from build123d import *

# Parameters (mm, degrees)
F1_DEPTH = 38.1
F2_DEPTH = 6.35
F0_W     = 6.3290558755
F0_H     = 12.5651992857
F3_DEPTH = 3.175
F0_R     = 8.6525424745
F0_R_2   = 9.0711492587
F0_W_2   = 5.1460258761
F0_H_2   = 10.5661942953
F0_W_3   = 24.5602354407
F0_W_4   = 26.5593226068
F0_W_5   = 6.9090700396
F0_W_6   = 14.06177961
F0_W_7   = 3.8753339521
F0_R_3   = 3.8842075561
F4_DEPTH = 25.4


with BuildPart() as f1:
    # F0 (on Front) → F1 (new body, symmetric)
    with BuildSketch(Plane.XZ):
        with BuildLine():
            Line((-51.1175096035, -16.873287037), (-51.1175096035, -22.5602444261))
            Line((-51.1175096035, -22.5602444261), (50.8410625258, -22.5602444261))
            ThreePointArc((50.8410625258, -22.5602444261), (83.7910011304, -14.7143733495), (109.6690327028, 7.1393135004))
            Line((109.6690327028, 7.1393135004), (93.1019932032, 7.1393135004))
            Line((93.1019932032, 7.1393135004), (71.9687715173, 7.1393135004))
            Line((71.9687715173, 7.1393135004), (50.8410625258, 7.1393135004))
            Line((50.8410625258, 7.1393135004), (45.6950366497, 7.1393135004))
            Line((45.6950366497, 7.1393135004), (21.134801209, 7.1393135004))
            Line((21.134801209, 7.1393135004), (-5.4245213978, 7.1393135004))
            Line((-5.4245213978, 7.1393135004), (-12.3335914374, 7.1393135004))
            Line((-12.3335914374, 7.1393135004), (-26.3953710475, 7.1393135004))
            Line((-26.3953710475, 7.1393135004), (-30.2707049996, 7.1393135004))
            Line((-30.2707049996, 7.1393135004), (-51.1175096035, 7.1393135004))
            Line((-51.1175096035, 7.1393135004), (-51.1175096035, 6.1453658742))
            Line((-51.1175096035, 6.1453658742), (-51.1175096035, -16.873287037))
        make_face()
    extrude(amount=F1_DEPTH, both=True)

    # F0 (on Front) → F2 (join, symmetric)
    with BuildSketch(Plane.XZ):
        Polygon((-55.0226159394, -16.873287037), (-51.1175096035, -16.873287037), (-51.1175096035, 6.1453658742), (-71.5858340263, 0), (-71.5858340263, -16.873287037), (-61.3516718149, -16.873287037), align=None)
    extrude(amount=F2_DEPTH, both=True)

    # F0 (on Front) → F3 (join, symmetric)
    with BuildSketch(Plane.XZ):
        with Locations((-58.1871438771, -23.1558866799)):
            Rectangle(F0_W, F0_H)
    extrude(amount=F3_DEPTH, both=True)

    # F0 (on Front) → F4 (join, symmetric)
    with BuildSketch(Plane.XZ):
        with BuildLine():
            Line((-30.2707049996, 50.5518508265), (-30.2707049996, 17.7055077956))
            Line((-30.2707049996, 17.7055077956), (-26.3953710475, 17.7055077956))
            Line((-26.3953710475, 17.7055077956), (-26.3953710475, 42.5316623055))
            add(Edge.make_bspline(
                [(-26.3953710475, 42.5316623055), (-25.6086271256, 50.5518508265), (-13.6145753786, 50.5218580365), (-12.3335914374, 42.5316623055)],
                knots=[0, 0, 0, 0, 14.06177961, 14.06177961, 14.06177961, 14.06177961], degree=3))
            Line((-12.3335914374, 42.5316623055), (-12.3335914374, 17.7055077956))
            Line((-12.3335914374, 17.7055077956), (-5.4245213978, 17.7055077956))
            Line((-5.4245213978, 17.7055077956), (21.134801209, 17.7055077956))
            Line((21.134801209, 17.7055077956), (45.6950366497, 17.7055077956))
            Line((45.6950366497, 17.7055077956), (50.8410625258, 17.7055077956))
            Line((50.8410625258, 17.7055077956), (50.8410625258, 50.5518508265))
            Line((50.8410625258, 50.5518508265), (-30.2707049996, 50.5518508265))
        make_face()
        with Locations((0, 36.2432263792)):
            Circle(F0_R, mode=Mode.SUBTRACT)
        with Locations((21.7964369804, 36.2432301044)):
            Circle(F0_R_2, mode=Mode.SUBTRACT)
        with Locations((48.2680495878, 12.422410648)):
            Rectangle(F0_W_2, F0_H_2)
        with Locations((33.4149189293, 12.422410648)):
            Rectangle(F0_W_3, F0_H_2)
        with Locations((7.8551399056, 12.422410648)):
            Rectangle(F0_W_4, F0_H_2)
        with Locations((-8.8790564176, 12.422410648)):
            Rectangle(F0_W_5, F0_H_2)
        with Locations((-19.3644812425, 12.422410648)):
            Rectangle(F0_W_6, F0_H_2)
        with Locations((-28.3330380235, 12.422410648)):
            Rectangle(F0_W_7, F0_H_2)
        with BuildLine():
            Line((-26.3953710475, 42.5316623055), (-26.3953710475, 17.7055077956))
            Line((-26.3953710475, 17.7055077956), (-12.3335914374, 17.7055077956))
            Line((-12.3335914374, 17.7055077956), (-12.3335914374, 42.5316623055))
            add(Edge.make_bspline(
                [(-26.3953710475, 42.5316623055), (-25.6086271256, 50.5518508265), (-13.6145753786, 50.5218580365), (-12.3335914374, 42.5316623055)],
                knots=[0, 0, 0, 0, 14.06177961, 14.06177961, 14.06177961, 14.06177961], degree=3))
        make_face()
        with Locations((-19.3260274827, 41.0979650915)):
            Circle(F0_R_3, mode=Mode.SUBTRACT)
        Polygon((-30.2707049996, 77.3901939392), (-30.2707049996, 50.5518508265), (50.8410625258, 50.5518508265), (44.1557221366, 52.7639029697), (16.5465753325, 61.8992451966), align=None)
    extrude(amount=F4_DEPTH, both=True)


solid = f1.part
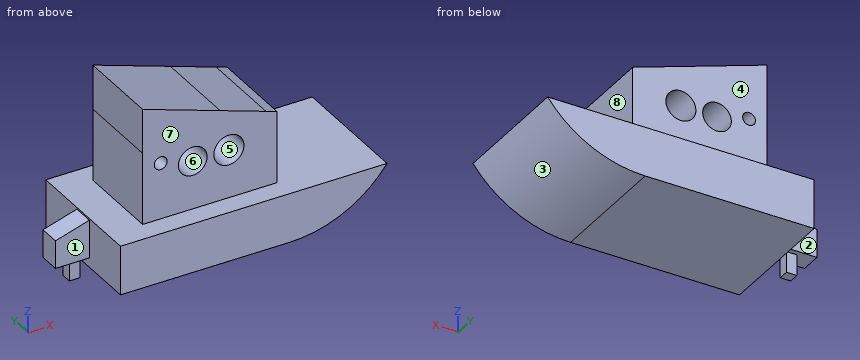
Model file for the job. Use its own axes, mm. Face numbers are marked on the shaded views. A direction names the side the tool comes from. Give positions to 0.01 mm unless a question says otherwise; leave off trailing zeros. Write each loop counter-clockwise with the first axis right and the second up, starting at its lowest first coordinate (ties: lowest second). Pieces come first, ordered by that corner, then holes. Notation, with made-up numbers: M 47,38.25 L 70,38.25 A29 ccw 70,58.25 Z; hole C 65,84 d9. An arc over 180 degrees is marked long. One line per item, written item: value. Start each with the question number.
Q1. Probe probe 1 along Z at (x, y) = (-40, 34); probe 2 along Y at (x, z) = (-20, 33); probe 3 along Z at (x, y) = (-61, 3.5). List the from-to ranges inside material, lowest first. Write a range as [from, to].
Q2. Saw through at C-C, the plane y = -15.5. Write the cut outline in (x, z), plus the area to 3 significant figures.
Q3. Saw through at D-D, the plane x = -38. Write the cut outline in (y, z), plus the area to 3 significant figures.
Q4. Two-plate mould, pull along X, no slides. Class the marked faces 6, 7 and 8: +X half, -X half, draft (parallel to the pull), parting line (faces both ways), or undercut.
Q5. Saw through at A-A, the plane x = 0. Write the cut outline in (y, z), plus the area to 3 significant figures.
Q6. Drop flat-ended pins along their axis: pin 1 Ø12 at (x, y) = (9, 3) entering from -Z; pin 2 Ø15 at (y, z) = (-16.5, -14.5) entering from -X; pin 3 Ø3 at (x, z) = (-58, -24.5) entering from +Y (3 decimals); pin 4 Ø14 at (x, z) = (0, 36.24) entering from -Y. Give the stop position or say it passes through.
Q7. 3-axis set-ups, long thin cutter, end or side, ignore diameter. For the marked faces 1, 2, 3, 4 and 5: which of +Z, -Z, +X, -X, +Y, -Y reach the whole face in a straight line?
Q8. Saw through at B-B, the plane z = -20. Write the cut outline in (x, y) (1 decimal).
Output values:
1. probe 1: z = [-22.56, 7.14]
1. probe 2: y = [-25.4, 25.4]
1. probe 3: z = [-16.87, 3.18]
2. outline: M -51.12,-22.56 L 50.84,-22.56 A73.11 ccw 109.67,7.14 L 50.84,7.14 L 50.84,50.55 L -30.27,77.39 L -30.27,7.14 L -51.12,7.14 Z; hole C -19.33,41.1 d7.77; hole C 0,36.24 d17.31; hole C 21.8,36.24 d18.14
2. area: 8,320 mm²
3. outline: M -38.1,-22.56 L 38.1,-22.56 L 38.1,7.14 L -38.1,7.14 Z
3. area: 2,260 mm²
4. face 6: undercut
4. face 7: draft
4. face 8: +X half
5. outline: M -38.1,-22.56 L 38.1,-22.56 L 38.1,7.14 L 25.4,7.14 L 25.4,27.59 L -25.4,27.59 L -25.4,7.14 L -38.1,7.14 Z; M -25.4,44.9 L 25.4,44.9 L 25.4,67.37 L -25.4,67.37 Z
5. area: 4,440 mm²
6. pin 1: stops at z = -22.56
6. pin 2: stops at x = -51.12
6. pin 3: stops at y = 3.175
6. pin 4: passes through
7. face 1: +Z, -Z, -X, -Y
7. face 2: +Z, -Z, -X, +Y
7. face 3: -Z, +X, +Y, -Y
7. face 4: +Z, +X, -X, +Y
7. face 5: +Y, -Y
8. outline: M -61.4,-3.2 L -55,-3.2 L -55,3.2 L -61.4,3.2 Z; M -51.1,-38.1 L 70,-38.1 L 70,38.1 L -51.1,38.1 Z
